Build history of the part. All positions in model axes, mm. Round coordinates to 2 decimals unless told otherwise and drop trailing zeros. Order: outer loops, then holes, each group sorted by start corner. A loop starts at its lowest first (then second) coordinate and runs counter-clockwise, first axis right, second up. Notation, with made-up numbers: M -13.75,-29 L 1.25,-29 A30 ccw 1.25,6 Z; hole C -21,-22 d8. An arc over 180 degrees is marked long. One line per question, with ' | ' between items. Start each with the question number.
Autodesk Inventor part; units mm, degrees
ref_plane "YZ Plane" through (0, 0, 0) normal (1, 0, 0) x (0, 1, 0)
ref_plane "XZ Plane" through (0, 0, 0) normal (0, 1, 0) x (-1, 0, 0)
ref_plane "XY Plane" through (0, 0, 0) normal (0, 0, 1) x (1, 0, 0)
sketch "Sketch1" plane through (0, 0, 0) normal (0, 0, 1) x (1, 0, 0)
  line L0 (117.475, 3.175) -> (117.475, -14.9225)
  line L1 (114.3, 3.175) -> (117.475, 3.175)
  line L2 (0, -14.9225) -> (-3.175, -14.9225)
  line L3 (0, -27.6225) -> (-3.175, -27.6225)
  line L4 (0, -14.9225) -> (0, -27.6225)
  line L5 (-3.175, -47.625) -> (-3.175, -27.6225)
  line L6 (-3.175, -14.9225) -> (-3.175, 3.175)
  line L7 (22.225, 0) -> (22.225, 3.175)
  line L8 (34.925, 0) -> (34.925, 3.175)
  line L9 (34.925, 0) -> (22.225, 0)
  line L10 (-3.175, 3.175) -> (22.225, 3.175)
  line L11 (79.375, 0) -> (79.375, 3.175)
  line L12 (92.075, 0) -> (92.075, 3.175)
  line L13 (92.075, 0) -> (79.375, 0)
  line L14 (34.925, 3.175) -> (79.375, 3.175)
  line L15 (92.075, 3.175) -> (117.475, 3.175)
  line L16 (114.3, -14.9225) -> (117.475, -14.9225)
  line L17 (114.3, -27.6225) -> (117.475, -27.6225)
  line L18 (114.3, -14.9225) -> (114.3, -27.6225)
  line L19 (117.475, 3.175) -> (117.475, -14.9225)
  line L20 (117.475, -27.6225) -> (117.475, -47.625)
  line L21 (92.075, -47.625) -> (92.075, -44.45)
  line L22 (92.075, -44.45) -> (79.375, -44.45)
  line L23 (79.375, -44.45) -> (79.375, -47.625)
  line L24 (22.225, -47.625) -> (22.225, -44.45)
  line L25 (22.225, -44.45) -> (34.925, -44.45)
  line L26 (34.925, -44.45) -> (34.925, -47.625)
  line L27 (22.225, -47.625) -> (-3.175, -47.625)
  line L28 (117.475, -47.625) -> (92.075, -47.625)
  line L29 (79.375, -47.625) -> (34.925, -47.625)
  point P0 (0, 0)
  dimension "d0" = 3.175
extrude "Extrusion1" add sketch "Sketch1" along normal blind 3.175
properties part number "top" material "ABS Plastic"
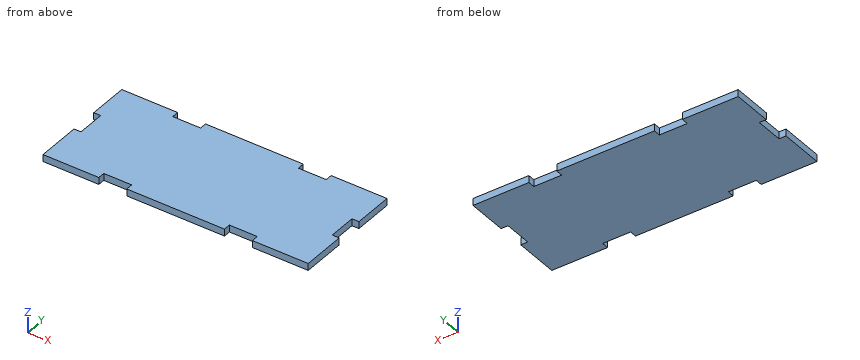
Item 1: Flat gauge pins, fed straight in: pin 1 (1.5 mm diameter, centred on x = 25.5, z = 2, fed in from +Y); pin 2 (5 mm diameter, centred on x = 77.5, y = -28.5, fed in from -Z); pin 3 (1 mm diameter, centred on y = -21, z = 2, fed in from +X). Where does each tip first touch, or does it go through?
Item 2: Wall check: line 1 along X through (y, z) = (-16, 1.8); line 2 along Y through (x, z) = (91.5, 0.95). Give the ranges that are in metal, low to high. Write a range as [from, to].
Item 3: Cut at B-B on y = -25.5. Write the cut outline in (x, z) (3 decimals).
Item 4: Cut at C-C on x = 27. Write the cut outline in (y, z) (3 decimals).
Results found:
1) pin 1: stops at y = 0 | pin 2: stops at z = 0 | pin 3: stops at x = 114.3
2) line 1: x = [0, 114.3] | line 2: y = [-44.45, 0]
3) outline: M 0,0 L 114.3,0 L 114.3,3.175 L 0,3.175 Z
4) outline: M -44.45,0 L 0,0 L 0,3.175 L -44.45,3.175 Z
